Build history of the part. All positions in model axes, mm. A direction names the side the tool comes from. Coordinates: 2 decimals unless noted, no trailing zeros. Loops run counter-clockwise (first coordinate to the right, second up) from the corner with the lowest first, then second, coordinate; pieces in that order, holes last. Notation, with made-up numbers: (78.5, -5) - (105.5, -5) arc R25 ccw to (105.5, 33) - close; hole circle Ø8 at (-10, -33). An arc over 180 degrees is marked (long way). One line per item, written item: value.
```python
from build123d import *

# Parameters (mm, degrees)
BOSS_EXTRUDE1_DEPTH = 1
BOSS_EXTRUDE2_DEPTH = 0.5
SKETCH3_R           = 1
BOSS_EXTRUDE3_DEPTH = 0.5
FILLET1_R           = 0.1
SKETCH4_W           = 7
SKETCH4_H           = 0.8
BOSS_EXTRUDE4_DEPTH = 0.2
FILLET2_R           = 0.1


with BuildPart() as part:
    # Sketch1 → Boss-Extrude1 (new body)
    with BuildSketch(Plane(origin=(0, 0, 0), x_dir=(1, 0, 0), z_dir=(0, 1, 0))):
        Polygon((-1.07, 2.57), (-2.57, 1.07), (-2.57, -1.07), (-1.07, -2.57), (1.07, -2.57), (2.57, -1.07), (2.57, 1.07), (1.07, 2.57), align=None)
    extrude(amount=BOSS_EXTRUDE1_DEPTH)

    # Sketch2 → Boss-Extrude2 (add)
    with BuildSketch(Plane(origin=(0, 1, 0), x_dir=(1, 0, 0), z_dir=(0, 1, 0))):
        Polygon((-1.77, 0.73862915), (-1.77, -0.73862915), (-0.73862915, -1.77), (0.73862915, -1.77), (1.77, -0.73862915), (1.77, 0.73862915), (0.73862915, 1.77), (-0.73862915, 1.77), align=None)
    extrude(amount=BOSS_EXTRUDE2_DEPTH)

    # Sketch3 → Boss-Extrude3 (add)
    with BuildSketch(Plane(origin=(0, 1.5, 0), x_dir=(1, 0, 0), z_dir=(0, 1, 0))):
        with Locations(Location((0, 0, 0), (0, 0, 270))):
            Circle(SKETCH3_R)
    extrude(amount=BOSS_EXTRUDE3_DEPTH)

    # Fillet1
    fillet1_edges = [part.edges().sort_by_distance(p)[0] for p in [
        (0, 1, 2.57),
        (1.82, 1, 1.82),
        (2.57, 1, 0),
        (1.82, 1, -1.82),
        (-1.254314575, 1, -1.254314575),
        (-1.77, 1, 0),
        (-1.254314575, 1, 1.254314575),
        (0, 1, -2.57),
        (0, 1, 1.77),
        (1.254314575, 1, 1.254314575),
        (1.77, 1, 0),
        (1.254314575, 1, -1.254314575),
        (0, 1, -1.77),
        (-1.254314575, 1.5, -1.254314575),
        (-1.77, 1.5, 0),
        (-1.254314575, 1.5, 1.254314575),
        (0, 1.5, 1.77),
        (1.254314575, 1.5, 1.254314575),
        (1.77, 1.5, 0),
        (1.254314575, 1.5, -1.254314575),
        (-1.82, 1, -1.82),
        (0, 1.5, -1.77),
        (0, 1.5, -1),
        (-2.57, 1, 0),
        (-1.82, 1, 1.82),
    ]]
    fillet(fillet1_edges, radius=FILLET1_R)

    # Sketch4 → Boss-Extrude4 (add)
    with BuildSketch(Plane.XZ):
        with Locations((0, 1.87)):
            Rectangle(SKETCH4_W, SKETCH4_H)
        with Locations((0, -1.87)):
            Rectangle(SKETCH4_W, SKETCH4_H)
    extrude(amount=-BOSS_EXTRUDE4_DEPTH)

    # Fillet2
    fillet2_edges = [part.edges().sort_by_distance(p)[0] for p in [
        (0, 2, -1),
    ]]
    fillet(fillet2_edges, radius=FILLET2_R)


solid = part.part
```
Item 1: Cut at A-A, the plane z = 0. Write the cut outline in (x, y), then the cut area to 3 significant figures.
Check result:
outline: (-2.57, 0) - (2.57, 0) - (2.57, 0.9) arc R0.1 ccw to (2.47, 1) - (1.87, 1) arc R0.1 cw to (1.77, 1.1) - (1.77, 1.4) arc R0.1 ccw to (1.67, 1.5) - (1.1, 1.5) arc R0.1 cw to (1, 1.6) - (1, 1.9) arc R0.1 ccw to (0.9, 2) - (-0.9, 2) arc R0.1 ccw to (-1, 1.9) - (-1, 1.6) arc R0.1 cw to (-1.1, 1.5) - (-1.67, 1.5) arc R0.1 ccw to (-1.77, 1.4) - (-1.77, 1.1) arc R0.1 cw to (-1.87, 1) - (-2.47, 1) arc R0.1 ccw to (-2.57, 0.9) - close
area: 7.91 mm^2
Item 2: Probe probe 1 along Z at (x, y) = (2.75, 0.15); probe 2 along Y at (x, z) = (1.25, -1.1); probe 3 along X at (y, z) = (0.6, -0.45). List the from-to ranges inside material, lowest first. Write a range as from..to.
Check result:
probe 1: z = -2.27..-1.47, 1.47..2.27
probe 2: y = 0..1.5
probe 3: x = -2.57..2.57
Item 3: Cut at D-D, the plane x = -2.25. Give the number of separate pieces and of enclosed holes in the cut face, then the cut area to 3 significant figures.
Check result:
separate pieces: 3
enclosed holes: 0
area: 3.09 mm^2
Item 4: Cut at C-C, the plane y = 0.6. Write the cut outline in (x, z).
Check result:
outline: (-2.57, -1.07) - (-1.07, -2.57) - (1.07, -2.57) - (2.57, -1.07) - (2.57, 1.07) - (1.07, 2.57) - (-1.07, 2.57) - (-2.57, 1.07) - close
Item 5: Cut at B-B, the plane x = 0. Write the cut outline in (y, z), then the cut area to 3 significant figures.
Check result:
outline: (0, -2.57) - (0.9, -2.57) arc R0.1 ccw to (1, -2.47) - (1, -1.87) arc R0.1 cw to (1.1, -1.77) - (1.4, -1.77) arc R0.1 ccw to (1.5, -1.67) - (1.5, -1.1) arc R0.1 cw to (1.6, -1) - (1.9, -1) arc R0.1 ccw to (2, -0.9) - (2, 0.9) arc R0.1 ccw to (1.9, 1) - (1.6, 1) arc R0.1 cw to (1.5, 1.1) - (1.5, 1.67) arc R0.1 ccw to (1.4, 1.77) - (1.1, 1.77) arc R0.1 cw to (1, 1.87) - (1, 2.47) arc R0.1 ccw to (0.9, 2.57) - (0, 2.57) - close
area: 7.91 mm^2
Item 6: Tool access for faces 4 (the face through (-3, 0.2, -2)), 5 (the face through (-1.26, 1.25, 1.25)), 6 (the face through (0, 0.4, 2.57)), 7 (the face through (1.26, 1.25, -1.25)), 8 (the face through (-2, 1, -1)): list every direction of +Z, -Z, +X, -X, +Y, -Y with a clear straight run to the whole face (end or side of a thin tool).
Check result:
face 4: -Z, -X, +Y
face 5: +Z, -X, +Y
face 6: +Z, +X, -X, +Y, -Y
face 7: -Z, +X, +Y
face 8: +Y
Item 7: Pull direction Z, two halves, no side cores. Call faces 1 (the face through (0, 2, 0)), 2 (the face through (2.57, 0.4, 0)), 3 (the face through (-1.25, 1.25, -1.26)): released by +Z, released by -Z, zero draft, split by the parting line, or undercut.
Check result:
face 1: zero draft
face 2: undercut
face 3: released by -Z
Item 8: Drop flat-ended pins along their axis: P1, Ø1, axis at y = 0, z = 0, coming from the -X side; P2, Ø3, axis at x = -1.5, z = -0.5, coming from the -Y side; P3, Ø0.7, axis at y = 0.5, z = -0.5, coming from the +X side; P4, Ø1.5, axis at x = 2.5, z = 1.5, coming from the +Y side. Give the stop position or say it passes through.
Check result:
P1: stops at x = -2.57
P2: stops at y = 0
P3: stops at x = 2.57
P4: stops at y = 1
